For this review, use the dimensioned drawing (mm, ordinates from the lowest corner) and the shaded views. A direction names the side the tool comes from. Coordinates: 2 decimals unless noted, no trailing zeros. Write each loop counter-clockwise with the first axis right and the second up, starting at its lowest first coordinate (ties: lowest second). Pieces come first, ordered by that corner, then holes. Notation, with made-up numbers: (-35, 8) - (9, 8) arc R29 ccw to (9, 43) - close; hole circle Ø4 at (37, 77). An arc over 180 degrees is marked (long way). Use one line per item in the form item = value. Start each with the question number.
1) Tool access review of the marked faces 1 and 2: name each direction out of +Z, -Z, +X, -X, +Y, -Y from which nothing blocks a thin tool from reaching the whole face with its end or side.
2) We need section D-D (z = 9). Give the boundary of the cut face in (x, y), plus the area to 3 significant figures.
3) Insertion check: P1, Ø5, axis at x = 7.5, y = 18, coming from the -Z side; P2, Ø1.2, axis at x = 27.5, y = 17.5, coming from the +Z side; P3, Ø3, axis at x = 7, y = 18.5, coming from the +Z side; P4, Ø5, axis at y = 15.5, z = 12.5, coming from the -X side. Each pin has a flat end and moves straight along its axis. Give the tip position at first contact, or say it passes through.
4) Mouldability with a two-part tool opening along Y and no side actions: class the marked faces 3, 4, 5 and 6 as pulls with the +Y half, pulls with the -Y half, needs draft (parallel to the pull), parting line crosses it, or undercut.
5) We need section B-B (x = 17.5). Give the boundary of the cut face in (y, z).
6) We need section C-C (y = 18). Give the boundary of the cut face in (x, z), plus the area to 3 significant figures.
7) For L1, parallel to Y at x = 27.5, z = 18.05; L2, parallel to Y at x = 9.5, z = 8.75; L3, parallel to X at y = 10.25, z = 9, list the stretches that pass through material, from the lowest coordinate up. Write a range as from..to.
8) We need section A-A (z = 17). Give the boundary of the cut face in (x, y), plus the area to 3 significant figures.
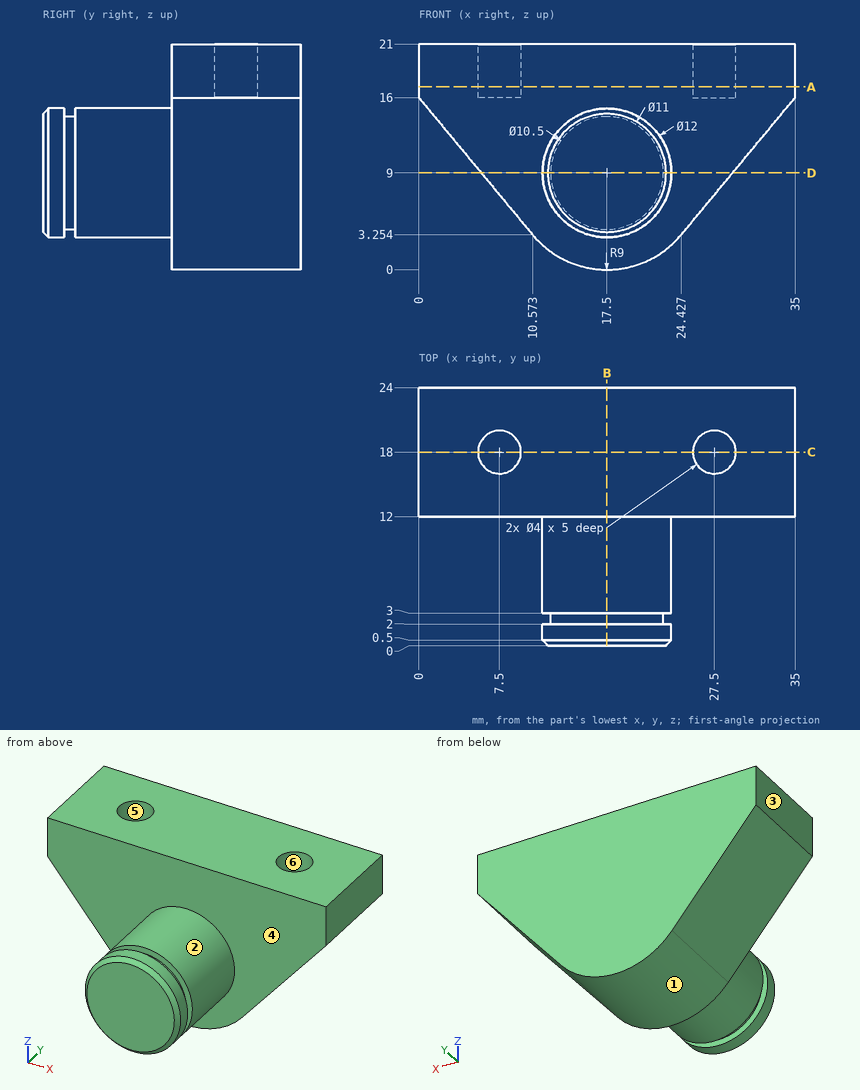
Determined:
q1.face_1 = -Z, +Y, -Y
q1.face_2 = -Y
q2.outline = (5.81, 12) - (11.5, 12) - (11.5, 3) - (12.25, 3) - (12.25, 2) - (11.5, 2) - (11.5, 0.5) - (12, 0) - (23, 0) - (23.5, 0.5) - (23.5, 2) - (22.75, 2) - (22.75, 3) - (23.5, 3) - (23.5, 12) - (29.19, 12) - (29.19, 24) - (5.81, 24) - close
q2.area = 423 mm²
q3.P1 = 3.94
q3.P2 = 16
q3.P3 = 21
q3.P4 = 0.83
q4.face_3 = needs draft
q4.face_4 = pulls with the -Y half
q4.face_5 = undercut
q4.face_6 = undercut
q5.outline = (0, 3.5) - (0.5, 3) - (2, 3) - (2, 3.75) - (3, 3.75) - (3, 3) - (12, 3) - (12, 0) - (24, 0) - (24, 21) - (12, 21) - (12, 15) - (3, 15) - (3, 14.25) - (2, 14.25) - (2, 15) - (0.5, 15) - (0, 14.5) - close
q6.outline = (0, 16) - (10.57, 3.25) arc R9 ccw to (24.43, 3.25) - (35, 16) - (35, 21) - (29.5, 21) - (29.5, 16) - (25.5, 16) - (25.5, 21) - (9.5, 21) - (9.5, 16) - (5.5, 16) - (5.5, 21) - (0, 21) - close
q6.area = 478 mm²
q7.L1 = 12..16, 20..24
q7.L2 = 12..24
q7.L3 = 11.5..23.5
q8.outline = (0, 12) - (35, 12) - (35, 24) - (0, 24) - close; hole circle Ø4 at (7.5, 18); hole circle Ø4 at (27.5, 18)
q8.area = 395 mm²
